```python
from build123d import *

# Parameters (mm, degrees)
CROQUIS1_R              = 2.1
SALIENTE_EXTRUIR1_DEPTH = 4
CROQUIS1_6_R            = 2.1
SALIENTE_EXTRUIR3_DEPTH = 5
REDONDEO1_R             = 1


with BuildPart() as part:
    # Croquis1 → Saliente-Extruir1 (new body)
    with BuildSketch(Plane.XY):
        with BuildLine():
            ThreePointArc((10, 54), (0, 64), (-10, 54))
            Line((-10, 54), (-10, -54))
            ThreePointArc((-10, -54), (0, -64), (10, -54))
            Line((10, -54), (10, 54))
        make_face()
        with Locations((0, 54)):
            Circle(CROQUIS1_R, mode=Mode.SUBTRACT)
        with BuildLine():
            Line((6, 38), (6, 22))
            Line((6, 22), (-6, 34))
            Line((-6, 34), (-6, 38))
            ThreePointArc((-6, 38), (0, 44), (6, 38))
        make_face(mode=Mode.SUBTRACT)
        Polygon((6, 16), (6, -16), (-6, -4), (-6, 4), align=None, mode=Mode.SUBTRACT)
        with BuildLine():
            Line((6, -22), (6, -38))
            ThreePointArc((6, -38), (0, -44), (-6, -38))
            Line((-6, -38), (-6, -34))
            Line((-6, -34), (6, -22))
        make_face(mode=Mode.SUBTRACT)
        Polygon((-6, -31), (-6, -7), (6, -19), align=None, mode=Mode.SUBTRACT)
        Polygon((-6, 7), (-6, 31), (6, 19), align=None, mode=Mode.SUBTRACT)
        with Locations((0, -54)):
            Circle(CROQUIS1_R, mode=Mode.SUBTRACT)
    extrude(amount=SALIENTE_EXTRUIR1_DEPTH)

    # Croquis1_6 → Saliente-Extruir3 (add)
    with BuildSketch(Plane.XY):
        with BuildLine():
            Line((10, 47.95), (10, 54))
            ThreePointArc((10, 54), (0, 64), (-10, 54))
            Line((-10, 54), (-10, 47.95))
            Line((-10, 47.95), (10, 47.95))
        make_face()
        with Locations((0, 54)):
            Circle(CROQUIS1_6_R, mode=Mode.SUBTRACT)
    extrude(amount=SALIENTE_EXTRUIR3_DEPTH)

    # Redondeo1
    redondeo1_edges = [part.edges().sort_by_distance(p)[0] for p in [
        (6, 22, 2),
        (-6, 34, 2),
        (6, -22, 2),
        (-6, -34, 2),
        (-6, -31, 2),
        (6, -19, 2),
        (-6, -7, 2),
        (-6, -4, 2),
        (6, -16, 2),
        (6, 16, 2),
        (-6, 4, 2),
        (-6, 7, 2),
        (6, 19, 2),
        (-6, 31, 2),
    ]]
    fillet(redondeo1_edges, radius=REDONDEO1_R)


solid = part.part
```
Verification items for the finished model (mm, model axes). A direction names the side the tool comes from. Round coordinates to 2 decimals unless told otherwise and drop trailing zeros. Order: outer loops, then holes, each group sorted by start corner. A loop starts at its lowest first (then second) coordinate and runs counter-clockwise, first axis right, second up. Notation, with made-up numbers: (-4.75, 28) - (44.25, 28) arc R29 ccw to (44.25, 65) - close; hole circle Ø10 at (-17, 10.5). An arc over 180 degrees is marked (long way). Use CSV: the item, a comma, the result in double quotes.
(1) Section check D-D on y = -41. Record the boundary of the cut face in (x, z), and give its area (3 significant figures).
Entries:
outline,"(-10, 0) - (-5.2, 0) - (-5.2, 4) - (-10, 4) - close; (5.2, 0) - (10, 0) - (10, 4) - (5.2, 4) - close"
area,"38.4 mm^2"
(2) Gauge pin test, flat ends, axial feed: pin 1 Ø1 at (x, z) = (3.5, 3) entering from -Y; pin 2 Ø10 at (x, y) = (3.5, 19) entering from +Z; pin 3 Ø2 at (x, z) = (7, 1) entering from -Y; pin 4 Ø8 at (x, y) = (-5, 23) entering from -Z. Record the tip position at first contact, or that the pin passes through.
Entries:
pin 1,"y = -63.54"
pin 2,"z = 4"
pin 3,"y = -62"
pin 4,"z = 0"
(3) Mould release check, pull along Y, two halves, no side actions. Record for faces 3 (the face through (0, -64, 2)), 4 (the face through (-6, 19, 2)), 5 (the face through (6, 0, 2)), 6 (the face through (-10, 1, 2)): released by +Y, released by -Y, zero draft, split by the parting line, or undercut.
Entries:
face 3,"released by -Y"
face 4,"undercut"
face 5,"undercut"
face 6,"zero draft"
(4) Thickness scan on probe 1 along X at (y, z) = (-36, 3.25); probe 2 along X at (y, z) = (-12, 3.6); probe 3 along X at (y, z) = (26.5, 1.05). Record the ranges inside material, lowest first. Write a range as from..to.
Entries:
probe 1,"-10..-6, 6..10"
probe 2,"-10..-6, -1..2, 6..10"
probe 3,"-10..-6, -1.5..1.5, 6..10"
(5) Section check B-B on y = -1. Record the boundary of the cut face in (x, z), and give its area (3 significant figures).
Entries:
outline,"(-10, 0) - (-6, 0) - (-6, 4) - (-10, 4) - close; (6, 0) - (10, 0) - (10, 4) - (6, 4) - close"
area,"32.0 mm^2"
(6) Access from +Z, -Z, +X, -X, +Y, -Y to the whole of each face (thin tool, end or side, straight path). Record for faces 1 (the face through (0, 25, 2)), 2 (the face through (-7, 1, 0)).
Entries:
face 1,"+Z, -Z"
face 2,"-Z, +X, -X, +Y, -Y"
(7) Section check A-A on x = 0. State how many separate pieces and enclosed holes the cut face has, and give its area (3 significant figures).
Entries:
separate pieces,"8"
enclosed holes,"0"
area,"186 mm^2"
